Work out the finished part from the listing and answer in its coordinate system (mm). A direction names the side the tool comes from. Coordinates: 2 decimals unless noted, no trailing zeros. Order: outer loops, then holes, each group sorted by start corner. A loop starts at its lowest first (then second) coordinate and runs counter-clockwise, first axis right, second up. Notation, with made-up numbers: (-7, 49.25) -> (30, 49.25) arc R17 ccw to (30, 75.25) -> close; hole circle Ø9 at (29, 41.25). An arc over 180 degrees is marked (long way). Answer as CSV lines item,"result". Start each with the question number.
Item 1: Which of the six approach directions +Z, -Z, +X, -X, +Y, -Y give full straight-line access (tool end or side, diameter ignored) to faces 1 (the face through (-68.5, -1, -10)), 2 (the face through (-33, 20.3, -11)), 3 (the face through (-69.49, 16.28, -2.97))?
Item 2: Section A-A (x = -5.5) is taken. Write down the section's boundary in (y, z).
Item 3: Section B-B (x = -61.5) is taken. Write down the section's boundary in (y, z).
Item 4: For a pull along X with two mould halves and no side action, classify faces 4 (the face through (-13, 0, -18.3)), 5 (the face through (2, 0, -10)), 6 (the face through (-33, -20.3, -11)) as pulls with the +X half, pulls with the -X half, needs draft (parallel to the pull), parting line crosses it, or undercut.
Item 5: Straight lines are drawn through the part: L1, parallel to X at y = -17, z = -7; L2, parallel to Y at x = -16, z = -9.5; L3, parallel to X at y = 0, z = -14.5. For each, find the intervals that lie inside material, in ascending order.
Item 6: Each of these flat-tipped pins is pushed along its axis until it touches: pin 1 Ø1.6 at (x, y) = (-69, -10) entering from +Z; pin 2 Ø1.5 at (x, y) = (-39, -12.5) entering from +Z. Where does it stop, or does it pass through?
```python
from build123d import *

# Parameters (mm, degrees)
BOSS_EXTRUDE1_DEPTH      = 2
BOSS_EXTRUDE1_DEPTH_BACK = 28.2
BOSS_EXTRUDE2_DEPTH      = 40.3
BOSS_EXTRUDE3_DEPTH      = 2
BOSS_EXTRUDE4_DEPTH      = 2
FILLET1_R                = 2
FILLET2_R                = 2


with BuildPart() as part:
    # Sketch1 → Boss-Extrude1 (new, two sides: drawn at the far end of the back side and taken through both)
    with BuildSketch(Plane.YZ.offset(-BOSS_EXTRUDE1_DEPTH_BACK)):
        Polygon((-18.3, -1.3), (-18.3, -18.3), (18.3, -18.3), (18.3, -1.3), (20.3, -1.3), (20.3, -20.3), (-20.3, -20.3), (-20.3, -1.3), align=None)
    extrude(amount=BOSS_EXTRUDE1_DEPTH + BOSS_EXTRUDE1_DEPTH_BACK)

    # Sketch2 → Boss-Extrude2 (add)
    with BuildSketch(Plane(origin=(-28.2, 0, 0), x_dir=(0, -1, 0), z_dir=(-1, 0, 0))):
        with BuildLine():
            Line((-18.3, -1.3), (-16.950221237, -1.3))
            ThreePointArc((-16.950221237, -1.3), (0, -17), (16.950221237, -1.3))
            Line((16.950221237, -1.3), (18.3, -1.3))
            Line((18.3, -1.3), (20.3, -1.3))
            Line((20.3, -1.3), (20.3, -20.3))
            Line((20.3, -20.3), (-20.3, -20.3))
            Line((-20.3, -20.3), (-20.3, -1.3))
            Line((-20.3, -1.3), (-18.3, -1.3))
        make_face()
    extrude(amount=BOSS_EXTRUDE2_DEPTH)

    # Sketch3 → Boss-Extrude3 (add)
    with BuildSketch(Plane.YZ.offset(2)):
        with BuildLine():
            Line((3.249615362, -1.3), (20.3, -1.3))
            Line((20.3, -1.3), (20.3, -20.3))
            Line((20.3, -20.3), (-20.3, -20.3))
            Line((-20.3, -20.3), (-20.3, -1.3))
            Line((-20.3, -1.3), (-3.249615362, -1.3))
            ThreePointArc((-3.249615362, -1.3), (0, -3.5), (3.249615362, -1.3))
        make_face()
    extrude(amount=BOSS_EXTRUDE3_DEPTH)

    # Sketch4 → Boss-Extrude4 (add)
    with BuildSketch(Plane(origin=(-68.5, 0, 0), x_dir=(0, -1, 0), z_dir=(-1, 0, 0))):
        with BuildLine():
            Line((-20.3, -1.3), (-20.3, -20.3))
            Line((-20.3, -20.3), (20.3, -20.3))
            Line((20.3, -20.3), (20.3, -1.3))
            Line((20.3, -1.3), (16.950221237, -1.3))
            ThreePointArc((16.950221237, -1.3), (16.829001324, -2.405143328), (16.63580476, -3.5))
            Line((16.63580476, -3.5), (4.749736835, -3.5))
            ThreePointArc((4.749736835, -3.5), (0, -5.9), (-4.749736835, -3.5))
            Line((-4.749736835, -3.5), (-16.63580476, -3.5))
            ThreePointArc((-16.63580476, -3.5), (-16.829001324, -2.405143328), (-16.950221237, -1.3))
            Line((-16.950221237, -1.3), (-20.3, -1.3))
        make_face()
    extrude(amount=BOSS_EXTRUDE4_DEPTH)

    # Fillet1
    fillet1_edges = [part.edges().sort_by_distance(p)[0] for p in [
        (-28.2, 0, -17),
    ]]
    fillet(fillet1_edges, radius=FILLET1_R)

    # Fillet2
    # the kernel refuses this fillet: 2 mm, written as the material it adds along each edge
    with BuildSketch(Plane(origin=(-68.5, -16.63580476, -3.5), x_dir=(0, -0.15316112796135575, 0.9882012289415578), z_dir=(-1, 0, 0))) as fillet2_piece_1:
        with BuildLine():
            CenterArc((1.714344809, 1.997127842), FILLET2_R, 188.810163249, 84.260829523)
            Line((-0.262057649, 1.690805586), (0, 0))
            ThreePointArc((0, 0), (0.91074568, -0.024413344), (1.82149136, 0))
        make_face()
    extrude(amount=2)
    with BuildSketch(Plane(origin=(-68.5, 16.63580476, -3.5), x_dir=(0, 0.15316112796135792, 0.9882012289415576), z_dir=(-1, 0, 0))) as fillet2_piece_2:
        with BuildLine():
            CenterArc((1.714344809, -1.997127842), FILLET2_R, 86.929007228, 84.260829523)
            Line((-0.262057649, -1.690805586), (0, 0))
            ThreePointArc((0, 0), (0.91074568, 0.024413344), (1.82149136, 0))
        make_face()
    extrude(amount=2)
    # the kernel refuses this fillet: 2 mm, written as the material it takes off along each edge
    with BuildSketch(Plane(origin=(-66.196895208, -4.749736835, -3.5), x_dir=(0, 0.6461838477214604, -0.7631817836819014), z_dir=(-1, 0, 0))) as fillet2_2_piece_1:
        with BuildLine():
            CenterArc((0.931071921, 1.995442745), FILLET2_R, 220.254494439, 45.876878938)
            Line((-0.595291646, 0.703075049), (0, 0))
            ThreePointArc((0, 0), (0.398066981, 0.013443903), (0.796133961, 0))
        make_face()
    extrude(amount=6.606209583, mode=Mode.SUBTRACT)
    with BuildSketch(Plane(origin=(-66.196895208, 4.749736835, -3.5), x_dir=(0, 1, 0), z_dir=(-1, 0, 0))) as fillet2_2_piece_2:
        with BuildLine():
            CenterArc((0.921241917, 2), FILLET2_R, 224.123121062, 45.876878938)
            ThreePointArc((-0.514448906, 0.607594937), (-0.246964311, 0.312484702), (0, 0))
            Line((0, 0), (0.921241917, 0))
        make_face()
    extrude(amount=6.606209583, mode=Mode.SUBTRACT)


solid = part.part
```
Checked values:
1,face 1,"+Z"
1,face 2,"+Z, -Z, +X, -X, +Y"
1,face 3,"+Z, -X"
2,outline,"(-20.3, -20.3) -> (20.3, -20.3) -> (20.3, -1.3) -> (18.3, -1.3) -> (18.3, -18.3) -> (-18.3, -18.3) -> (-18.3, -1.3) -> (-20.3, -1.3) -> close"
3,outline,"(-20.3, -20.3) -> (20.3, -20.3) -> (20.3, -1.3) -> (16.95, -1.3) arc R17 cw to (-16.95, -1.3) -> (-20.3, -1.3) -> close"
4,face 4,"undercut"
4,face 5,"undercut"
4,face 6,"needs draft"
5,L1,"x = -70.5 to -28.3, 2 to 4"
5,L2,"y = -20.3 to -18.3, 18.3 to 20.3"
5,L3,"x = -70.5 to -68.5, 2 to 4"
6,pin 1,"stops at z = -3.5"
6,pin 2,"stops at z = -10.65"
